```python
from build123d import *

# Parameters (mm, degrees)
SKETCH027_R         = 19.5
PAD014_DEPTH        = 10
HOLE004_D           = 3.25
HOLE004_DEPTH       = 55
HOLE004_CBORE_D     = 4
HOLE004_CBORE_DEPTH = 30
POCKET003_DEPTH     = 4
SKETCH033_W         = 2
SKETCH033_H         = 10
POCKET004_DEPTH     = 12
CHAMFER005_SIZE     = 2


with BuildPart() as part:
    # Sketch027 → Pad014 (new body)
    with BuildSketch(Plane.XZ.offset(85)):
        with BuildLine():
            Line((-27.5, 6), (-27.5, 13.999999))
            Line((-27.5, 13.999999), (-11.973302, 13.999999))
            ThreePointArc((11.973302, 13.999999), (0, 58.8), (-11.973302, 13.999999))
            Line((27.5, 13.999999), (11.973302, 13.999999))
            Line((27.5, 6), (27.5, 13.999999))
            Line((15.75, 6), (27.5, 6))
            Line((15.75, 6), (15.75, 0))
            Line((15.75, 0), (-15.75, 0))
            Line((-15.75, 6), (-15.75, 0))
            Line((-15.75, 6), (-27.5, 6))
        make_face()
        with Locations((0, 34.8)):
            Circle(SKETCH027_R, mode=Mode.SUBTRACT)
    extrude(amount=PAD014_DEPTH)

    # Hole004
    with Locations(Plane.XY.offset(50)):
        with Locations((-23, -90), (23, -90)):
            CounterBoreHole(HOLE004_D / 2, HOLE004_CBORE_D / 2, HOLE004_CBORE_DEPTH, depth=HOLE004_DEPTH)

    # Sketch029 → Pocket003 (cut)
    with BuildSketch(Plane.XY.offset(6)):
        Polygon((-21.412287, -92.75), (-19.824574, -90), (-21.412287, -87.25), (-24.587713, -87.25), (-26.175426, -90), (-24.587713, -92.75), align=None)
        Polygon((24.587713, -92.75), (26.175426, -90), (24.587713, -87.25), (21.412287, -87.25), (19.824574, -90), (21.412287, -92.75), align=None)
    extrude(amount=POCKET003_DEPTH, mode=Mode.SUBTRACT)

    # Sketch033 → Pocket004 (cut)
    with BuildSketch(Plane.XZ.offset(84)):
        with Locations((0, 57)):
            Rectangle(SKETCH033_W, SKETCH033_H)
    extrude(amount=POCKET004_DEPTH, mode=Mode.SUBTRACT)

    # Chamfer005
    chamfer005_edges = [part.edges().sort_by_distance(p)[0] for p in [
        (27.5, -85, 10),
        (-27.5, -85, 10),
        (0, -85, 0),
        (14.137716, -85, 48.230376),
        (-13.430376, -85, 20.662284),
        (11.973302, -90, 13.999999),
        (-11.973302, -90, 13.999999),
        (27.5, -95, 10),
        (-27.5, -95, 10),
        (0, -95, 0),
        (-1, -90, 58.779158),
        (1, -90, 58.779158),
    ]]
    chamfer(chamfer005_edges, length=CHAMFER005_SIZE)


solid = part.part
```
Design review of the part built by this model. Coordinates are the model's own, in mm. A direction names the side the tool comes from. Round coordinates to 2 decimals unless told otherwise and drop trailing zeros. Write each loop counter-clockwise with the first axis right and the second up, starting at its lowest first coordinate (ties: lowest second). Pieces come first, ordered by that corner, then holes. Notation, with made-up numbers: (78.5, 52) -> (106.5, 52) arc R11 cw to (106.5, 60) -> close; hole circle Ø4 at (-36, -12.75). An arc over 180 degrees is marked (long way). Write item = value, one per line. Start each with the question number.
1) Wall thickness on probe 1 along X at (y, z) = (-90, 11.75) (3 decimals); probe 2 along X at (y, z) = (-93, 34.8); probe 3 along Z at (x, y) = (17.5, -94): over which ranges is each line inside the solid? List them lowest first. Write a range as from..to.
2) Tool access review of faces 4 (the face through (-20, -91, 6)), 5 (the face through (-1, -90, 56)), 6 (the face through (5.8, -85, 13.7)), 7 (the face through (23, -92.75, 8)), 8 (the face through (0, -94, 1)): name each direction out of +Z, -Z, +X, -X, +Y, -Y from which nothing blocks a thin tool from reaching the whole face with its end or side.
3) Take a section at C-C, the plane y = -86. State the section outline as (x, z) points, plus the area to 3 significant figures.
4) Take a section at A-A, the plane x = 23. State the section outline as (y, z) points (3 decimals), plus the area to 3 significant figures.
5) Mouldability with a two-part tool opening along Y and no side actions: class faces 1 (the face through (21, -90, 35)), 2 (the face through (4, -95, 14)), 3 (the face through (20, -91, 6)) as +Y half, -Y half, draft (parallel to the pull), parting line (faces both ways), or undercut.
6) Clearance check with flat-ended pins moving along their axes: pin 1 (0.8 mm diameter, centred on y = -91, z = 55.5, fed in from -X); pin 2 (5 mm diameter, centred on x = 7.5, z = 50.5, fed in from +Y); pin 3 (2 mm diameter, centred on y = -90.5, z = 55, fed in from +X); pin 4 (6 mm diameter, centred on y = -87.5, z = 16.5, fed in from +X). State where each tip first meets the part, or that it passes through.
7) Take a section at B-B, the plane x = 0. State the section outline as (y, z) points.
Results list:
q1.probe_1 = -27.5..-24.625, -21.375..21.375, 24.625..27.5
q1.probe_2 = -24..-19.5, 19.5..24
q1.probe_3 = 6..14, 18.38..26.2, 43.4..51.22
q2.face_4 = -Z, -X, +Y, -Y
q2.face_5 = +Z, +Y, -Y
q2.face_6 = +Z, -Z, +X, -X, +Y
q2.face_7 = -Z
q2.face_8 = -Z, +X, -X, -Y
q3.outline = (-26.5, 6) -> (-15.75, 6) -> (-15.75, 1) -> (15.75, 1) -> (15.75, 6) -> (26.5, 6) -> (26.5, 14) -> (13.97, 14) -> (13.66, 15.07) arc R24 ccw to (2.99, 58.61) -> (1, 56.78) -> (1, 55.28) arc R20.5 cw (long way) to (-1, 55.28) -> (-1, 56.78) -> (-2.99, 58.61) arc R24 ccw to (-13.66, 15.07) -> (-13.97, 14) -> (-26.5, 14) -> close
q3.area = 1,010 mm²
q4.outline = (-95, 6) -> (-92.75, 6) -> (-92.75, 10) -> (-91.625, 10) -> (-91.625, 14) -> (-95, 14) -> close; (-95, 27.944) -> (-92, 27.944) -> (-92, 41.656) -> (-95, 41.656) -> close; (-88.375, 10) -> (-87.25, 10) -> (-87.25, 6) -> (-85, 6) -> (-85, 14) -> (-88.375, 14) -> close; (-88, 27.944) -> (-85, 27.944) -> (-85, 41.656) -> (-88, 41.656) -> close
q4.area = 127 mm²
q5.face_1 = undercut
q5.face_2 = -Y half
q5.face_3 = draft
q6.pin_1 = -12.8
q6.pin_2 = -86.6
q6.pin_3 = 14.4
q6.pin_4 = 27.5
q7.outline = (-95, 2) -> (-93, 0) -> (-87, 0) -> (-85, 2) -> (-85, 13.3) -> (-87, 15.3) -> (-95, 15.3) -> close
